Can you work these out from the model? Positions are in its coordinate system, mm. Give positions to 0.01 mm unless a question says otherwise; leave off trailing zeros. Loops run counter-clockwise (first coordinate to the right, second up) from the corner with the lowest first, then second, coordinate; pieces in that order, holes last. Notation, with made-up numbers: (62, -24.5) - (85, -24.5) arc R16 cw to (85, -13.5) - close; hole circle Ø5 at (31.5, 55.25). An arc over 180 degrees is marked (long way). Answer as a JSON object with one key per item and string values.
```python
from build123d import *

# Parameters (mm, degrees)
PAD001_DEPTH = 1016
SKETCH_R     = 3.96875
POCKET_DEPTH = 6.35


with BuildPart() as part:
    # Sketch004 → Pad001 (new body, symmetric)
    with BuildSketch(Plane.YZ):
        Polygon((-12.7, 14.789829), (-12.7, 24.977896), (12.7, 24.977896), (12.7, 14.789829), (14.325, 14.789829), (14.325, 26.566591), (-14.325, 26.566591), (-14.325, 14.789829), align=None)
    extrude(amount=PAD001_DEPTH, both=True)

    # Sketch (on Face6 of Pad001) → Pocket (cut)
    with BuildSketch(Plane(origin=(0, 0, 26.566591), x_dir=(0, -1, 0), z_dir=(0, 0, 1))):
        with Locations((0, 990.6)):
            Circle(SKETCH_R)
    pocket = extrude(amount=-POCKET_DEPTH, mode=Mode.SUBTRACT)

    # Mirrored: Pocket across Sketch H_Axis
    add(pocket.mirror(Plane(origin=(0, 0, 26.566591), x_dir=(0, 0, 1), z_dir=(1, 0, 0))), mode=Mode.SUBTRACT)


with BuildPart() as part_1:
    # Body001 placement: moved
    add(part.part.moved(Location((0, 0, 19.05))))


solid = part_1.part
```
1) Imagine slicing it at A-A on x = -549.5. Write out the boundary of the cut face in (y, z) (3 decimals), and give its area (3 significant figures).
Check sheet entries:
{"outline": "(-14.325, 33.84) - (-12.7, 33.84) - (-12.7, 44.028) - (12.7, 44.028) - (12.7, 33.84) - (14.325, 33.84) - (14.325, 45.617) - (-14.325, 45.617) - close", "area": "78.6 mm2"}
2) I need wall thicknesses on L1, parallel to X at y = 0, z = 44.85; L2, parallel to Y at x = 269, z = 40.25 (3 decimals); L3, parallel to Y at x = 990.6, z = 44.7 (3 decimals). Which ranges of each line are inside material? Lowest first, please.
Check sheet entries:
{"L1": "-1016 to -994.57, -986.63 to 986.63, 994.57 to 1016", "L2": "-14.325 to -12.7, 12.7 to 14.325", "L3": "-14.325 to -3.969, 3.969 to 14.325"}
3) Imagine slicing it at B-B on z = 39.25. Write out the boundary of the cut face in (x, y) (3 decimals).
Check sheet entries:
{"outline": "(-1016, -14.325) - (1016, -14.325) - (1016, -12.7) - (-1016, -12.7) - close; (-1016, 12.7) - (1016, 12.7) - (1016, 14.325) - (-1016, 14.325) - close"}
4) I'm going to push a flat-ended pin straight in: P1, Ø9, axis at x = 990.6, y = 0, coming from the -Z side. Where does the tip first touch, or does it pass through?
Check sheet entries:
{"P1": "z = 44.03"}
